Autodesk Inventor part; units mm, degrees
ref_plane "YZ Plane" through (0, 0, 0) normal (1, 0, 0) x (0, 1, 0)
ref_plane "XZ Plane" through (0, 0, 0) normal (0, 1, 0) x (-1, 0, 0)
ref_plane "XY Plane" through (0, 0, 0) normal (0, 0, 1) x (1, 0, 0)
sketch "Sketch1" plane through (0, 0, 0) normal (0, 0, 1) x (1, 0, 0)
  line L0 (8.25, 4.95) -> (-8.25, 4.95)
  line L1 (-8.25, 4.95) -> (-8.25, -4.95)
  line L2 (-8.25, -4.95) -> (8.25, -4.95)
  line L3 (8.25, -4.95) -> (8.25, 4.95)
  point P0 (0, 0)
  dimension "d19" = 9.9
extrude "Box" add sketch "Sketch1" along normal mid plane 12.446
sketch "Sketch3" plane through (0, 0, -6.223) normal (0, 0, -1) x (-1, 0, 0)
  line L0 (-5.08, 0) -> (5.08, 0) construction
  line L1 (-4.75, 0) -> (4.75, 0) construction
  line L2 (-2.972, -1.778) -> (2.972, -1.778)
  line L3 (2.972, 1.778) -> (-2.972, 1.778)
  arc A0 (-2.972, 1.778) -> (-2.972, -1.778) centre (-2.972, 0) ccw
  arc A1 (2.972, -1.778) -> (2.972, 1.778) centre (2.972, 0) ccw
  point P0 (0, 0)
  point P1 (0, 0)
  point P2 (0, 0)
  dimension "d31" = 9.5
extrude "Slot" cut sketch "Sketch3" against normal blind 10.16
sketch "Sketch4" plane through (0, 0, -6.223) normal (0, 0, -1) x (-1, 0, 0)
  circle A0 centre (-2.5426, 3.364) radius 1.2
  line L0 (-2.972, 1.778) -> (2.972, 1.778)
  line L1 (8.25, 4.95) -> (-8.25, 4.95)
  point P0 (0, 0)
  dimension "d32" = 2.4
  dimension "d33" = 3.172
  dimension "d34" = 1.586
extrude "MountingHole" cut sketch "Sketch4" against normal blind 12.5
pattern_linear "Mounting Holes" count 2 spacing 5.92 along (-1, 0, 0) count 2 spacing 6.648 along (0, -1, 0) of "MountingHole"
sketch "Sketch6" plane through (-8.25, 4.95, 6.223) normal (0, 1, 0) x (1, 0, 0)
  circle A0 centre (8.25, 7.366) radius 1.105
  point P0 (8.25, 6.223)
  dimension "d20" = 2.21
extrude "CentralSMAHole" cut sketch "Sketch6" against normal blind 10
sketch "Sketch8" plane through (-8.25, 4.95, 6.223) normal (0, 1, 0) x (1, 0, 0)
  circle A0 centre (14.36, 7.366) radius 1.295
  point P0 (8.25, 6.223)
  dimension "d23" = 2.59
extrude "SMAMounting" cut sketch "Sketch8" against normal blind 10
pattern_linear "SMAMountingHoles" count 2 spacing 12.22 along (-1, 0, 0) of "SMAMounting"
equation "\"d34\" = 0.5 * d33"
properties part number "NewSink"
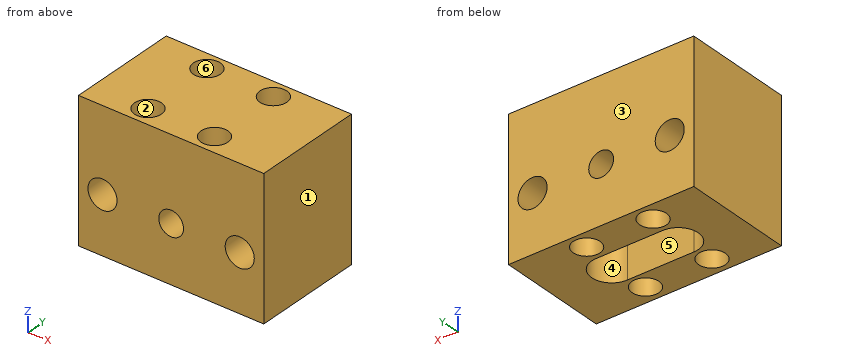
Geometry: final body of the model. Coordinates: model frame, mm. Face numbers are marked on the shaded views. A direction names the side the tool comes from. Round coordinates to 2 decimals unless told otherwise and drop trailing zeros. Loops run counter-clockwise (first coordinate to the right, second up) from the corner with the lowest first, then second, coordinate; pieces in that order, holes last.
Q1. Section B-B on x = 0. Return loops of the section in (y, z), plus the area to 3 significant figures.
Q2. Material intervals for L1, parallel to X at y = 3.25, z = -4.25; L2, parallel to X at y = -2.5, z = 3.25; L3, parallel to X at y = -3.5, z = -0.25, sorted ascending.
Q3. Pin query (flat end, axial travel): P1, Ø2, axis at x = 0, z = -1.143, coming from the -Y side; P2, Ø6.5, axis at x = -0.5, z = -2, coming from the +Y side. Return the tip coordinate at first contact, or that it passes through.
Q4. Section D-D on z = 5.75. Return loops of the section in (x, y).
Q5. Section A-A on z = -1.75. Return loops of the section in (x, y).
Q6. Section C-C on x = -6.11. Return loops of the section in (y, z), plus the area to 3 significant figures.
Q7. Pull-direction query (X, two-part tool) for the marked faces 1, 2, 3 and 4; classes: released by +X, released by -X, zero draft, split by the parting line, or undercut.
Q8. Access query for the marked faces 5 and 6. Directions: +Z, -Z, +X, -X, +Y, -Y. A direction counts if a zero-diameter tool reaches every point of the face in a straight line with its end or side. Return the directions, or none.
Evaluation:
1. outline: (-4.95, -6.22) - (-1.78, -6.22) - (-1.78, -2.25) - (-4.95, -2.25) - close; (-4.95, -0.04) - (-1.78, -0.04) - (-1.78, 3.94) - (1.78, 3.94) - (1.78, -0.04) - (4.95, -0.04) - (4.95, 6.22) - (-4.95, 6.22) - close; (1.78, -6.22) - (4.95, -6.22) - (4.95, -2.25) - (1.78, -2.25) - close
1. area: 73.1 mm2
2. L1: x = -8.25 to -4.57, -2.18 to 1.35, 3.74 to 8.25
2. L2: x = -8.25 to -4.29, -2.47 to 1.63, 3.45 to 8.25
2. L3: x = -8.25 to -7.05, -5.17 to -4.56, -2.2 to -0.65, 0.65 to 1.36, 3.72 to 5.17, 7.05 to 8.25
3. P1: passes through
3. P2: stops at y = 4.95
4. outline: (-8.25, -4.95) - (8.25, -4.95) - (8.25, 4.95) - (-8.25, 4.95) - close; hole circle Ø2.4 at (-3.38, -3.28); hole circle Ø2.4 at (-3.38, 3.36); hole circle Ø2.4 at (2.54, -3.28); hole circle Ø2.4 at (2.54, 3.36)
5. outline: (-8.25, -4.95) - (-7.25, -4.95) - (-7.25, 4.95) - (-8.25, 4.95) - close; (-4.97, -4.95) - (-0.92, -4.95) - (-0.92, -1.78) - (-2.97, -1.78) arc R1.78 cw to (-2.97, 1.78) - (-0.92, 1.78) - (-0.92, 4.95) - (-4.97, 4.95) - close; (0.92, -4.95) - (4.97, -4.95) - (4.97, 4.95) - (0.92, 4.95) - (0.92, 1.78) - (2.97, 1.78) arc R1.78 cw to (2.97, -1.78) - (0.92, -1.78) - close; (7.25, -4.95) - (8.25, -4.95) - (8.25, 4.95) - (7.25, 4.95) - close; hole circle Ø2.4 at (-3.38, -3.28); hole circle Ø2.4 at (-3.38, 3.36); hole circle Ø2.4 at (2.54, -3.28); hole circle Ø2.4 at (2.54, 3.36)
6. outline: (-4.95, -6.22) - (4.95, -6.22) - (4.95, -2.44) - (-4.95, -2.44) - close; (-4.95, 0.15) - (4.95, 0.15) - (4.95, 6.22) - (-4.95, 6.22) - close
6. area: 97.6 mm2
7. face 1: released by +X
7. face 2: undercut
7. face 3: zero draft
7. face 4: undercut
8. face 5: -Z
8. face 6: +Z, -Z
